Read the model definition and answer for the solid it produces. Units are mm, in the model's axes. Coordinates: 2 decimals unless noted, no trailing zeros. Write each loop counter-clockwise with the first axis right and the second up, starting at its lowest first coordinate (ties: lowest second). Pieces come first, ordered by that corner, then holes.
(1) Section B-B on x = 85 is taken. Write down the section's boundary in (y, z), then the cut area to 3 significant figures.
(2) Given pin 1 (10 mm diameter, centred on x = 91, y = -11, fed in from -Z); pin 2 (10 mm diameter, centred on x = 85, y = -10, fed in from +Z), each flat-ended and moving along its own axis, determine where each tip first touches the part or whether it passes through.
(3) Section A-A on z = 53 is taken. Write down the section's boundary in (x, y), then the cut area to 3 significant figures.
(4) Find the intervals of material crossed by probe 1 along X at (y, z) = (-14.5, 43); probe 2 along Y at (x, z) = (85, 6.5), in increasing order.
(5) Section C-C on y = -3.75 is taken. Write down the section's boundary in (x, z), then the cut area to 3 significant figures.
(6) Section D-D on y = -10 is taken. Write down the section's boundary in (x, z), then the cut area to 3 significant figures.
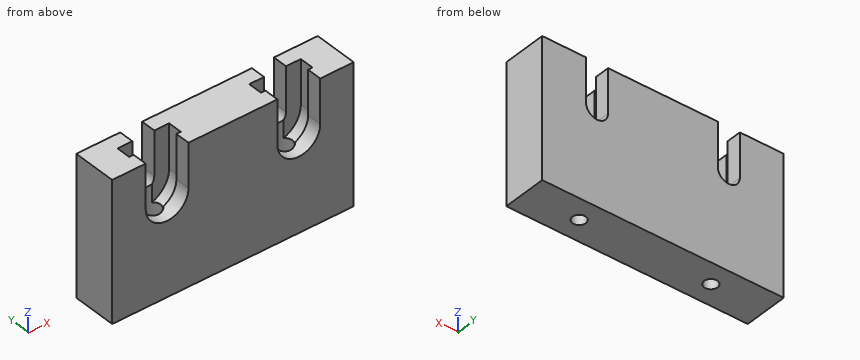
from build123d import *

# Parameters (mm, degrees)
F0_W      = 110
F0_H      = 63.25
F1_DEPTH  = 20
F2_R      = 9.75
F3_DEPTH  = 6.75
F4_R      = 11.75
F5_DEPTH  = 6.5
F6_R      = 5
F7_DEPTH  = 6.75
F8_W      = 19.5
F8_H      = 20
F9_DEPTH  = 6.75
F10_W     = 23.5
F10_H     = 20
F11_DEPTH = 6.5
F12_W     = 10
F12_H     = 20
F13_DEPTH = 6.75
F14_R     = 5.1
F15_DEPTH = 50
F16_R     = 3.05
F17_DEPTH = 13.25


with BuildPart() as f1:
    # F0 (on Front) → F1 (new body)
    with BuildSketch(Plane.XZ):
        with Locations((55, 31.625)):
            Rectangle(F0_W, F0_H)
    extrude(amount=F1_DEPTH)

    # F2 (on face) → F3 (cut)
    with BuildSketch(Plane.XZ.offset(20)):
        with Locations((25, 43.25)):
            Circle(F2_R)
        with Locations((85, 43.25)):
            Circle(F2_R)
    extrude(amount=-F3_DEPTH, mode=Mode.SUBTRACT)

    # F4 (on face) → F5 (cut)
    with BuildSketch(Plane.XZ.offset(13.25)):
        with Locations((25, 43.25)):
            Circle(F4_R)
        with Locations((85, 43.25)):
            Circle(F4_R)
    extrude(amount=-F5_DEPTH, mode=Mode.SUBTRACT)

    # F6 (on face) → F7 (cut, through all)
    with BuildSketch(Plane.XZ.offset(6.75)):
        with Locations((25, 43.25)):
            Circle(F6_R)
        with Locations((85, 43.25)):
            Circle(F6_R)
    extrude(amount=-F7_DEPTH, mode=Mode.SUBTRACT)

    # F8 (on face) + F6 (on face) → F9 (cut)
    with BuildSketch(Plane.XZ.offset(20)):
        with Locations((25, 53.25)):
            Rectangle(F8_W, F8_H)
        with Locations((85, 53.25)):
            Rectangle(F8_W, F8_H)
    with BuildSketch(Plane.XZ.offset(6.75)):
        with Locations((25, 43.25)):
            Circle(F6_R)
        with Locations((85, 43.25)):
            Circle(F6_R)
    extrude(amount=-F9_DEPTH, mode=Mode.SUBTRACT)

    # F10 (on face) → F11 (cut)
    with BuildSketch(Plane.XZ.offset(13.25)):
        with Locations((25, 53.25)):
            Rectangle(F10_W, F10_H)
        with Locations((85, 53.25)):
            Rectangle(F10_W, F10_H)
    extrude(amount=-F11_DEPTH, mode=Mode.SUBTRACT)

    # F12 (on face) → F13 (cut, through all)
    with BuildSketch(Plane.XZ.offset(6.75)):
        with Locations((25, 53.25)):
            Rectangle(F12_W, F12_H)
        with Locations((85, 53.25)):
            Rectangle(F12_W, F12_H)
    extrude(amount=-F13_DEPTH, mode=Mode.SUBTRACT)

    # F14 (on face) → F15 (cut)
    with BuildSketch(Plane.XY.offset(63.25)):
        with Locations((25, -10)):
            Circle(F14_R)
        with Locations((85, -10)):
            Circle(F14_R)
    extrude(amount=-F15_DEPTH, mode=Mode.SUBTRACT)

    # F16 (on face) → F17 (cut, through all)
    with BuildSketch(Plane(origin=(0, 0, 0), x_dir=(1, 0, 0), z_dir=(0, 0, -1))):
        with Locations((25, 10)):
            Circle(F16_R)
        with Locations((85, 10)):
            Circle(F16_R)
    extrude(amount=-F17_DEPTH, mode=Mode.SUBTRACT)


solid = f1.part
Response:
1. outline: (-20, 0) - (-13.05, 0) - (-13.05, 13.25) - (-15.1, 13.25) - (-15.1, 33.5) - (-20, 33.5) - close; (-6.95, 0) - (0, 0) - (0, 38.25) - (-4.9, 38.25) - (-4.9, 13.25) - (-6.95, 13.25) - close
1. area: 406 mm2
2. pin 1: stops at z = 0
2. pin 2: stops at z = 13.25
3. outline: (0, -20) - (15.25, -20) - (15.25, -13.25) - (13.25, -13.25) - (13.25, -6.75) - (20, -6.75) - (20, 0) - (0, 0) - close; (30, -6.75) - (36.75, -6.75) - (36.75, -13.25) - (34.75, -13.25) - (34.75, -20) - (75.25, -20) - (75.25, -13.25) - (73.25, -13.25) - (73.25, -6.75) - (80, -6.75) - (80, 0) - (30, 0) - close; (90, -6.75) - (96.75, -6.75) - (96.75, -13.25) - (94.75, -13.25) - (94.75, -20) - (110, -20) - (110, 0) - (90, 0) - close
3. area: 1,500 mm2
4. probe 1: x = 0 to 15.25, 34.75 to 75.25, 94.75 to 110
4. probe 2: y = -20 to -13.05, -6.95 to 0
5. outline: (0, 0) - (110, 0) - (110, 63.25) - (90, 63.25) - (90, 43.25) arc R5 cw to (80, 43.25) - (80, 63.25) - (30, 63.25) - (30, 43.25) arc R5 cw to (20, 43.25) - (20, 63.25) - (0, 63.25) - close
5. area: 6,480 mm2
6. outline: (0, 0) - (21.95, 0) - (21.95, 13.25) - (19.9, 13.25) - (19.9, 32.66) arc R11.75 cw to (13.25, 43.25) - (13.25, 63.25) - (0, 63.25) - close; (28.05, 0) - (81.95, 0) - (81.95, 13.25) - (79.9, 13.25) - (79.9, 32.66) arc R11.75 cw to (73.25, 43.25) - (73.25, 63.25) - (36.75, 63.25) - (36.75, 43.25) arc R11.75 cw to (30.1, 32.66) - (30.1, 13.25) - (28.05, 13.25) - close; (88.05, 0) - (110, 0) - (110, 63.25) - (96.75, 63.25) - (96.75, 43.25) arc R11.75 cw to (90.1, 32.66) - (90.1, 13.25) - (88.05, 13.25) - close
6. area: 5,040 mm2
